Autodesk Inventor part; units mm, degrees
ref_plane "Start Plane" through (0, 0, 0) normal (0, 0, 1) x (1, 0, 0)
ref_plane "End Plane" through (0, 0, 700) normal (0, 0, 1) x (1, 0, 0)
ref_plane "YZ Plane" through (0, 0, 0) normal (1, 0, 0) x (0, 1, 0)
ref_plane "Start Plane" through (0, 0, 0) normal (0, 0, 1) x (1, 0, 0)
ref_plane "End Plane" through (0, 0, 700) normal (0, 0, 1) x (1, 0, 0)
sketch "Sketch" plane through (0, 0, 0) normal (0, 0, 1) x (1, 0, 0)
  line L0 (-12.5, -25) -> (12.5, -25)
  line L1 (12.5, -25) -> (12.5, 25)
  line L2 (12.5, 25) -> (-12.5, 25)
  line L3 (-12.5, 25) -> (-12.5, -25)
  line L4 (-12.5, -25) -> (12.5, 25) construction
  line L5 (12.5, -25) -> (-12.5, 25) construction
  line L6 (-9.5, 22) -> (9.5, 22)
  line L7 (9.5, 22) -> (9.5, -22)
  line L8 (9.5, -22) -> (-9.5, -22)
  line L9 (-9.5, -22) -> (-9.5, 22)
  point P0 (0, 0)
  dimension "Width" = 25
  dimension "Height" = 50
  dimension "Thickness" = 3
extrude "Body" add sketch "Sketch" along normal up to surface (700 mm away) from surface at 0
sketch "Sketch2" plane through (0, 0, 0) normal (0, 0, 1) x (1, 0, 0)
  line L0 (0, 0) -> (10, 0)
ref_plane "Work Plane3" through (0, 0, 0) normal (0, -1, 0) x (1, 0, 0)
sketch "Sketch3" plane through (0, 0, 0) normal (0, -1, 0) x (1, 0, 0)
  line L0 (-2, 0) -> (12, 0)
  line L1 (-2, 700) -> (12, 700)
  dimension "d10" = 700
equation "\"G_OFFSET_START\" = 0"
equation "\"G_OFFSET_END\" = 0"
equation "\"G_L\" = 100"
properties part number "25x50x3" material "Aluminum 6061"
Geometry check sheet. Reference: the model listing, model coordinates, mm. A direction names the side the tool comes from. Give positions to 0.01 mm unless a question says otherwise; leave off trailing zeros. Loops run counter-clockwise (first coordinate to the right, second up) from the corner with the lowest first, then second, coordinate; pieces in that order, holes last. Notation, with made-up numbers: (88, -32.75) -> (93, -32.75) arc R18 cw to (93, -12.75) -> close; hole circle Ø8 at (-21, 74). An arc over 180 degrees is marked (long way). Answer in a Markdown table with one row per item. Add a question column.
1) Cross-section at C-C on z = 276. Record the boundary of the cut face in (x, y), and give its area (3 significant figures).
2) Material ranges on probe 1 along X at (y, z) = (20.5, 671); probe 2 along Y at (x, z) = (2.5, 290), recorded low to high. Write a range as from..to.
3) Draft check along X on faces 1 (the face through (12.5, 0, 345)), 2 (the face through (-12.5, 0, 345)), 3 (the face through (-9.5, 0, 345)), 4 (the face through (0, 25, 345)). Enter one of: pulls with the +X half, pulls with the -X half, needs draft (parallel to the pull), parting line crosses it, or undercut.
4) Set-up check for faces 5 (the face through (9.5, 0, 345)), 6 (the face through (-10, -2, 0)): record each of +Z, -Z, +X, -X, +Y, -Y from which the full face is reachable in a straight line by a thin tool's end or side.
5) Cross-section at A-A on x = -2. Record the boundary of the cut face in (y, z).
6) Cross-section at B-B on y = -0.5. Record the boundary of the cut face in (x, z).
Outcome:
| question | item | result |
|---|---|---|
| 1 | outline | (-12.5, -25) -> (12.5, -25) -> (12.5, 25) -> (-12.5, 25) -> close; hole (-9.5, -22) -> (9.5, -22) -> (9.5, 22) -> (-9.5, 22) -> close |
| 1 | area | 414 mm^2 |
| 2 | probe 1 | x = -12.5..-9.5, 9.5..12.5 |
| 2 | probe 2 | y = -25..-22, 22..25 |
| 3 | face 1 | pulls with the +X half |
| 3 | face 2 | pulls with the -X half |
| 3 | face 3 | undercut |
| 3 | face 4 | needs draft |
| 4 | face 5 | +Z, -Z |
| 4 | face 6 | -Z, +X, -X, +Y, -Y |
| 5 | outline | (-25, 0) -> (-22, 0) -> (-22, 700) -> (-25, 700) -> close; (22, 0) -> (25, 0) -> (25, 700) -> (22, 700) -> close |
| 6 | outline | (-12.5, 0) -> (-9.5, 0) -> (-9.5, 700) -> (-12.5, 700) -> close; (9.5, 0) -> (12.5, 0) -> (12.5, 700) -> (9.5, 700) -> close |
